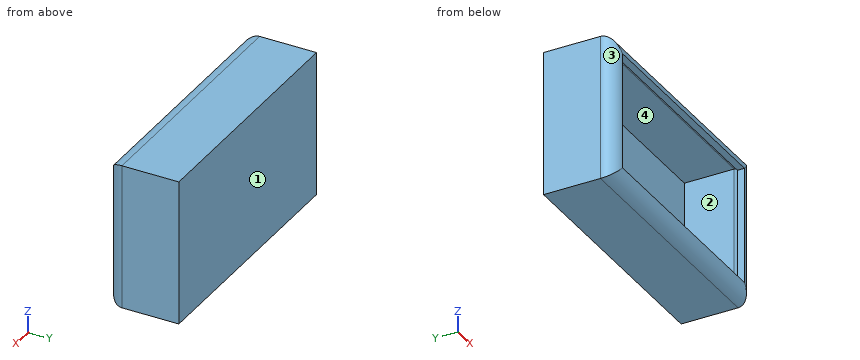
```python
from build123d import *

# Parameters (mm, degrees)
F0_W     = 88
F0_H     = 51.0847450688
F1_DEPTH = 25
F2_R     = 5
F3_T     = -2.5


# Not quite as in the source:
# - a shell that OpenCascade refuses in one call is made with other operations: the cavity is built on its own and cut out


with BuildPart() as f1:
    # F0 (on Front) → F1 (new body)
    with BuildSketch(Plane.XZ):
        with Locations((-8.0169501303, 25.5423725344)):
            Rectangle(F0_W, F0_H)
    extrude(amount=F1_DEPTH)

    # F2
    f2_edges = [f1.edges().sort_by_distance(p)[0] for p in [
        (-52.01695, -25, 25.542373),
        (-8.01695, -25, 0),
        (35.98305, -25, 25.542373),
        (-8.01695, -25, 51.084745),
    ]]
    fillet(f2_edges, radius=F2_R)

    # F3: a shell. OpenCascade refuses it in one call, so the cavity is built on its own and cut out:
    # the body offset inwards by the wall thickness, plus a prism from it out through each open face.
    f3_core = offset(f1.part, amount=F3_T, mode=Mode.PRIVATE)
    f3_exits = [f3_core.faces().sort_by_distance(p)[0] for p in [
        (-8.01695, -22.5, 25.542373),
    ]]
    add(f3_core, mode=Mode.SUBTRACT)
    extrude(f3_exits, amount=-F3_T, mode=Mode.SUBTRACT)


solid = f1.part
```
The model under review builds one solid part; all positions refer to its coordinate system, in mm. Face numbers are marked on the shaded views. Round coordinates to 2 decimals unless told otherwise and drop trailing zeros. Loops run counter-clockwise (first coordinate to the right, second up) from the corner with the lowest first, then second, coordinate; pieces in that order, holes last.
Item 1: Take a section at B-B (x = -18). Write out the cut boundary in (y, z), then the cut area to 3 significant figures.
Determined:
outline: (-25, 5) arc R5 ccw to (-20, 0) - (0, 0) - (0, 51.08) - (-20, 51.08) arc R5 ccw to (-25, 46.08) - (-22.5, 46.08) arc R2.5 cw to (-20, 48.58) - (-2.5, 48.58) - (-2.5, 2.5) - (-20, 2.5) arc R2.5 cw to (-22.5, 5) - close
area: 245 mm2
Item 2: Clearance check with flat-ended pins moving along their axes: pin 1 Ø2 at (x, z) = (18.5, 12) entering from +Y; pin 2 Ø1.2 at (x, y) = (8, -24) entering from -Z; pin 3 Ø3 at (x, z) = (10, 37.5) entering from -Y; pin 4 Ø0.8 at (y, z) = (-23.5, 30.5) entering from -X. State where each tip first meets the part, or that it passes through.
Determined:
pin 1: stops at y = 0
pin 2: stops at z = 1.33
pin 3: stops at y = -2.5
pin 4: stops at x = -50.94
Item 3: For line 1 (Z direction, x = 9.5, y = -18.5); line 2 (X direction, y = -11, z = 28.5); line 3 (Y direction, x = -14, z = 7), list the stretches that pass through material, from the lowest coordinate up.
Determined:
line 1: z = 0 to 2.5, 48.58 to 51.08
line 2: x = -52.02 to -49.52, 33.48 to 35.98
line 3: y = -2.5 to 0
Item 4: Take a section at A-A (y = -12.5). Write out the cut boundary in (x, z), then the cut area to 3 significant figures.
Determined:
outline: (-52.02, 0) - (35.98, 0) - (35.98, 51.08) - (-52.02, 51.08) - close; hole (-49.52, 2.5) - (33.48, 2.5) - (33.48, 48.58) - (-49.52, 48.58) - close
area: 670 mm2
Item 5: Mouldability with a two-part tool opening along Y and no side actions: class the marked faces 1, 2, 3 and 4 as released by +Y, released by -Y, zero draft, split by the parting line, or undercut.
Determined:
face 1: released by +Y
face 2: undercut
face 3: released by -Y
face 4: undercut
Item 6: Take a section at C-C (z = 43.5). Write out the cut boundary in (x, y).
Determined:
outline: (-52.02, -20) arc R5 ccw to (-47.02, -25) - (-47.02, -22.5) arc R2.5 cw to (-49.52, -20) - (-49.52, -2.5) - (33.48, -2.5) - (33.48, -20) arc R2.5 cw to (30.98, -22.5) - (30.98, -25) arc R5 ccw to (35.98, -20) - (35.98, 0) - (-52.02, 0) - close
